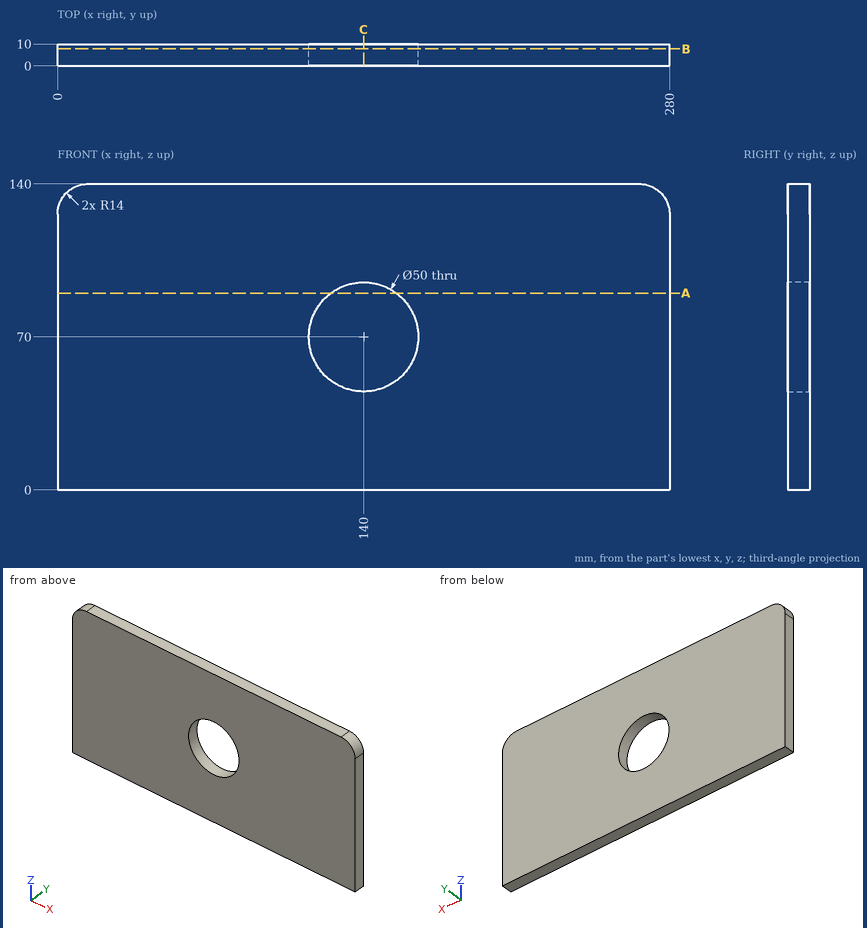
Source: three-view drawing plus pictorial views. Frame: mm from the lowest corner of the part. Give positions to 0.01 mm unless a question says otherwise; leave off trailing zeros. Order: outer loops, then holes, each group sorted by start corner. A loop starts at its lowest first (then second) coordinate and runs counter-clockwise, first axis right, second up. Notation, with made-up numbers: (12, -11.75) -> (64, -11.75) arc R27 cw to (64, 25.25) -> close; hole circle Ø4 at (29.25, -39.5). An arc over 180 degrees is marked (long way). Put each result on its own line as item: value.
Q1. Section B-B, the plane y = 7.75. Return loops of the section in (x, z), then the cut area to 3 significant figures.
Here are the results:
outline: (0, 0) -> (280, 0) -> (280, 126) arc R14 ccw to (266, 140) -> (14, 140) arc R14 ccw to (0, 126) -> close; hole circle Ø50 at (140, 70)
area: 37,200 mm^2
Q2. Section C-C, the plane x = 140. Return loops of the section in (y, z).
Here are the results:
outline: (0, 0) -> (10, 0) -> (10, 45) -> (0, 45) -> close; (0, 95) -> (10, 95) -> (10, 140) -> (0, 140) -> close
Q3. Section A-A, the plane z = 90. Return loops of the section in (x, y).
Here are the results:
outline: (0, 0) -> (125, 0) -> (125, 10) -> (0, 10) -> close; (155, 0) -> (280, 0) -> (280, 10) -> (155, 10) -> close
Q4. Material intervals for L1, parallel to X at y = 7.75, z = 70; L2, parallel to X at y = 5.25, z = 55.5; L3, parallel to Z at x = 142, y = 9.5, sorted ascending.
Here are the results:
L1: x = 0 to 115, 165 to 280
L2: x = 0 to 119.63, 160.37 to 280
L3: z = 0 to 45.08, 94.92 to 140
